The model under review builds one solid part; all positions refer to its coordinate system, in mm. A direction names the side the tool comes from. Coordinates: 2 decimals unless noted, no trailing zeros. Write each loop counter-clockwise with the first axis right and the second up, starting at its lowest first coordinate (ties: lowest second). Pieces come first, ordered by that corner, then holes.
Autodesk Inventor part; units mm, degrees
ref_plane "YZ Plane" through (0, 0, 0) normal (1, 0, 0) x (0, 1, 0)
ref_plane "XZ Plane" through (0, 0, 0) normal (0, 1, 0) x (-1, 0, 0)
ref_plane "XY Plane" through (0, 0, 0) normal (0, 0, 1) x (1, 0, 0)
sketch "Sketch1" plane through (0, 0, 0) normal (0, 0, 1) x (1, 0, 0)
  point P0 (0, 0)
sketch "Sketch2" plane through (0, 0, 0) normal (0, 0, 1) x (1, 0, 0)
  line L0 (0, 0) -> (250, 0)
  line L1 (250, 0) -> (250, 250)
  line L2 (250, 250) -> (0, 250)
  line L3 (0, 250) -> (0, 0)
  line L4 (0, 0) -> (-70, 0)
  line L5 (-70, 0) -> (0, 70)
  dimension "d0" = 250
  dimension "d1" = 250
  dimension "d2" = 70
  dimension "d3" = 45
extrude "Extrusion1" add sketch "Sketch2" along normal blind 142
sketch "Sketch3" plane through (0, 0, 142) normal (0, 0, 1) x (1, 0, 0)
  line L0 (4, 3) -> (180, 3)
  line L1 (-70, 0) -> (250, 0)
  line L2 (4, 3) -> (180, 3) construction
  line L3 (180, 3) -> (180, 246)
  line L4 (4, 3) -> (4, 246)
  line L5 (4, 3) -> (247, 3) construction
  line L6 (250, 250) -> (0, 250)
  line L7 (4, 246) -> (180, 246)
  point P0 (0, 0)
  dimension "d6" = 176
  dimension "d7" = 0
  dimension "d8" = 243
  dimension "d9" = 243
  dimension "d10" = 90
extrude "Extrusion2" cut sketch "Sketch3" against normal blind 135
sketch "Sketch4" plane through (4, 3, 142) normal (0, 1, 0) x (1, 0, 0)
  line L0 (3, 3) -> (173, 3)
  line L1 (176, 0) -> (0, 0)
  line L2 (173, 3) -> (173, 132)
  line L3 (173, 132) -> (3, 132)
  line L4 (176, 135) -> (0, 135)
  line L5 (3, 132) -> (3, 3)
  line L6 (176, 0) -> (176, 135)
  line L7 (0, 0) -> (0, 135)
  point P0 (-4, 142)
  dimension "d13" = 3
  dimension "d14" = 3
  dimension "d15" = 3
  dimension "d16" = 3
extrude "Extrusion3" cut sketch "Sketch4" against normal through all contours L5 L3 L2 L0
sketch "Sketch5" plane through (4, 3, 142) normal (0, 1, 0) x (1, 0, 0)
  line L0 (176, 0) -> (0, 0)
  line L1 (0, 0) -> (0, 3)
  line L2 (3, 3) -> (3, 132)
  line L3 (0, 3) -> (176, 3)
  line L4 (176, 0) -> (176, 135)
  line L5 (176, 0) -> (0, 0)
  line L6 (3, 3) -> (173, 3)
  point P0 (-4, 142)
extrude "Extrusion4" add sketch "Sketch5" along normal blind 7
Item 1: Mouldability with a two-part tool opening along Z and no side actions: class faces 4 (the face through (91, 246, 75)), 5 (the face through (91, 5, 139)), 6 (the face through (186, 106, 142)) as pulls with the +Z half, pulls with the -Z half, needs draft (parallel to the pull), parting line crosses it, or undercut.
Solved:
face 4: needs draft
face 5: undercut
face 6: pulls with the +Z half
Item 2: Take a section at A-A, the plane x = 168. Write out the cut boundary in (y, z), plus the area to 3 significant figures.
Solved:
outline: (0, 0) - (250, 0) - (250, 142) - (246, 142) - (246, 7) - (3, 7) - (3, 10) - (0, 10) - close; (0, 139) - (10, 139) - (10, 142) - (0, 142) - close
area: 2,330 mm2
Item 3: For pin 1 (1.5 mm diameter, centred on y = 168.5, z = 78, fed in from -X); pin 2 (0.9 mm diameter, centred on y = 1, z = 106, fed in from -X); pin 3 (10 mm diameter, centred on x = 167.5, z = 26, fed in from -Y), all flat-tipped, find the tip position at first contact; note any pin that passes through.
Solved:
pin 1: stops at x = 0
pin 2: stops at x = -69.45
pin 3: stops at y = 246
Item 4: Machinability: for faces 1 (the face through (0, 161, 70)), 2 (the face through (127, 250, 70)), 3 (the face through (52.5, 3, 9.8)), which of the approach directions +Z, -Z, +X, -X, +Y, -Y give a long, thin tool a straight path to every point of the face, cutting with its end or side? Answer none if there is none.
Solved:
face 1: +Z, -Z, -X, +Y
face 2: +Z, -Z, +X, -X, +Y
face 3: none
Item 5: Take a section at D-D, the plane y = 62. Write out the cut boundary in (x, z).
Solved:
outline: (-8, 0) - (250, 0) - (250, 142) - (180, 142) - (180, 7) - (4, 7) - (4, 142) - (-8, 142) - close
Item 6: To check wall thickness, follow line 1 along X through (y, z) = (199.5, 10); line 2 along Y through (x, z) = (110.5, 117.5); line 3 along Z through (x, y) = (102.5, 54). State the ranges of each line that lie inside material, in increasing order.
Solved:
line 1: x = 0 to 4, 180 to 250
line 2: y = 246 to 250
line 3: z = 0 to 7
Item 7: Take a section at C-C, the plane z = 39.5. Write out the cut boundary in (x, y), plus the area to 3 significant figures.
Solved:
outline: (-70, 0) - (7, 0) - (7, 3) - (4, 3) - (4, 246) - (180, 246) - (180, 3) - (177, 3) - (177, 0) - (250, 0) - (250, 250) - (0, 250) - (0, 70) - close
area: 21,700 mm2
Item 8: Take a section at B-B, the plane y = 30.5. Write out the cut boundary in (x, z), plus the area to 3 significant figures.
Solved:
outline: (-39.5, 0) - (250, 0) - (250, 142) - (180, 142) - (180, 7) - (4, 7) - (4, 142) - (-39.5, 142) - close
area: 17,300 mm2
